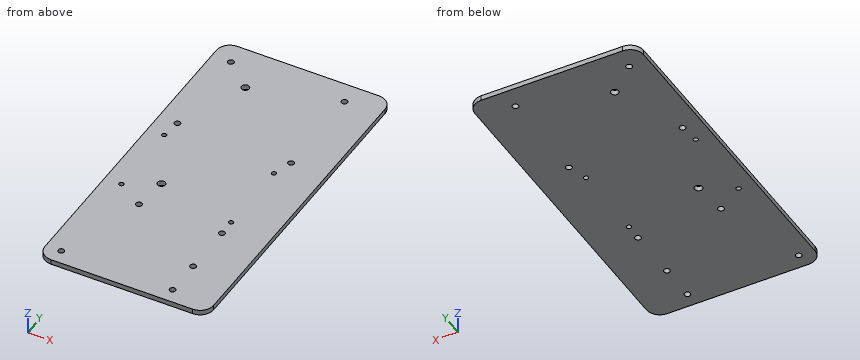
from build123d import *

# Parameters (mm, degrees)
CYLINDER_R        = 1.8
CYLINDER_DEPTH    = 10
CYLINDER002_R     = 2.3
CYLINDER002_DEPTH = 20
ARRAY001_Y_COUNT  = 2
ARRAY001_Y_PITCH  = 90
CYLINDER001_R     = 1.4
CYLINDER001_DEPTH = 10
ARRAY_X_COUNT     = 2
ARRAY_X_PITCH     = 65
ARRAY_Y_COUNT     = 2
ARRAY_Y_PITCH     = 46
CYLINDER011_R     = 1.8
CYLINDER011_DEPTH = 20
ARRAY007_X_COUNT  = 2
ARRAY007_X_PITCH  = 67.4
ARRAY007_Y_COUNT  = 2
ARRAY007_Y_PITCH  = 57.4
BOX_W             = 100
BOX_H             = 200
BOX_DEPTH         = 3
FILLET_R          = 8


with BuildPart() as m3_bolt_hole:
    # Cylinder → Cylinder (new body)
    with BuildSketch(Plane.XY):
        Circle(CYLINDER_R)
    extrude(amount=CYLINDER_DEPTH)


with BuildPart() as m3_bolt_hole_clone003:
    # Body003 base: copy of m3 bolt hole
    add(m3_bolt_hole.part)


with BuildPart() as m3_bolt_hole_clone003_1:
    # Body003 placement: moved
    add(m3_bolt_hole_clone003.part.moved(Location((30.2, -3.5, 0))))


with BuildPart() as m3_bolt_hole_clone002:
    # Body002 base: copy of m3 bolt hole
    add(m3_bolt_hole.part)


with BuildPart() as m3_bolt_hole_clone002_1:
    # Body002 placement: moved
    add(m3_bolt_hole_clone002.part.moved(Location((30.2, 27.5, 0))))


with BuildPart() as m3_bolt_hole_clone001:
    # Body001 base: copy of m3 bolt hole
    add(m3_bolt_hole.part)


with BuildPart() as m3_bolt_hole_clone001_1:
    # Body001 placement: moved
    add(m3_bolt_hole_clone001.part.moved(Location((-35.8, -25.5, 0))))


with BuildPart() as m3_bolt_hole_clone:
    # Body base: copy of m3 bolt hole
    add(m3_bolt_hole.part)


with BuildPart() as m3_bolt_hole_clone_1:
    # Body placement: moved
    add(m3_bolt_hole_clone.part.moved(Location((-19, 27.5, 0))))


with BuildPart() as attach_m4_bolt_array:
    # Cylinder002 → Cylinder002 (new body)
    with BuildSketch(Plane.XY):
        Circle(CYLINDER002_R)
    extrude(amount=CYLINDER002_DEPTH)

    # Array001 Y: attach m4 bolt array ×2


with BuildPart() as attach_m4_bolt_array_1:
    add(attach_m4_bolt_array.part)
    with Locations(*[(0, i * ARRAY001_Y_PITCH, 0) for i in range(1, ARRAY001_Y_COUNT)]):
        add(attach_m4_bolt_array.part)


with BuildPart() as attach_m4_bolt_array_2:
    # Array001 placement: moved
    add(attach_m4_bolt_array_1.part.moved(Location((-17, 48, -6))))


with BuildPart() as m2_5_bolt_hole_7x5_pcb_array:
    # Cylinder001 → Cylinder001 (new body)
    with BuildSketch(Plane.XY):
        Circle(CYLINDER001_R)
    extrude(amount=CYLINDER001_DEPTH)

    # Array X: m2.5 bolt hole 7x5 pcb array ×2


with BuildPart() as m2_5_bolt_hole_7x5_pcb_array_1:
    add(m2_5_bolt_hole_7x5_pcb_array.part)
    with Locations(*[(i * ARRAY_X_PITCH, 0, 0) for i in range(1, ARRAY_X_COUNT)]):
        add(m2_5_bolt_hole_7x5_pcb_array.part)

    # Array Y: m2.5 bolt hole 7x5 pcb array ×2


with BuildPart() as m2_5_bolt_hole_7x5_pcb_array_2:
    add(m2_5_bolt_hole_7x5_pcb_array_1.part)
    with Locations(*[(0, i * ARRAY_Y_PITCH, 0) for i in range(1, ARRAY_Y_COUNT)]):
        add(m2_5_bolt_hole_7x5_pcb_array_1.part)


with BuildPart() as m2_5_bolt_hole_7x5_pcb_array_3:
    # Array placement: moved
    add(m2_5_bolt_hole_7x5_pcb_array_2.part.moved(Location((-35, 37.6, 0))))


with BuildPart() as wall_box_hole_stand_array002:
    # Cylinder011 → Cylinder011 (new body)
    with BuildSketch(Plane(origin=(3.3, 3.3, 0), x_dir=(1, 0, 0), z_dir=(0, 0, 1))):
        Circle(CYLINDER011_R)
    extrude(amount=CYLINDER011_DEPTH)

    # Array007 X: wall box hole stand array002 ×2


with BuildPart() as wall_box_hole_stand_array002_1:
    add(wall_box_hole_stand_array002.part)
    with Locations(*[(i * ARRAY007_X_PITCH, 0, 0) for i in range(1, ARRAY007_X_COUNT)]):
        add(wall_box_hole_stand_array002.part)

    # Array007 Y: wall box hole stand array002 ×2


with BuildPart() as wall_box_hole_stand_array002_2:
    add(wall_box_hole_stand_array002_1.part)
    with Locations(*[(0, i * ARRAY007_Y_PITCH, 0) for i in range(1, ARRAY007_Y_COUNT)]):
        add(wall_box_hole_stand_array002_1.part)


with BuildPart() as wall_box_hole_stand_array002_3:
    # Array007 placement: moved
    add(wall_box_hole_stand_array002_2.part.moved(Location((-37, 92, -6))))


with BuildPart() as cnc_v4_m3_hole_fusion:
    # Body004 base: copy of m3 bolt hole
    add(m3_bolt_hole.part)


with BuildPart() as cnc_v4_m3_hole_fusion_1:
    # Body004 placement: moved
    add(cnc_v4_m3_hole_fusion.part.moved(Location((30.2, -25.5, 0))))

    # Fusion: union m3 bolt hole clone003, m3 bolt hole clone002, m3 bolt hole clone001, m3 bolt hole clone, attach m4 bolt array, m2.5 bolt hole 7x5 pcb array, wall box hole stand array002
    add(m3_bolt_hole_clone003_1.part)
    add(m3_bolt_hole_clone002_1.part)
    add(m3_bolt_hole_clone001_1.part)
    add(m3_bolt_hole_clone_1.part)
    add(attach_m4_bolt_array_2.part)
    add(m2_5_bolt_hole_7x5_pcb_array_3.part)
    add(wall_box_hole_stand_array002_3.part)


with BuildPart() as cnc_v4_m3_hole_fusion_2:
    # Fusion placement: moved
    add(cnc_v4_m3_hole_fusion_1.part.moved(Location((45, 34.4, -2.25))))


with BuildPart() as cnc_v4_plate_cut:
    # Box → Box (new body)
    with BuildSketch(Plane.XY):
        with Locations((50, 100)):
            Rectangle(BOX_W, BOX_H)
    extrude(amount=BOX_DEPTH)

    # Fillet
    fillet_edges = [cnc_v4_plate_cut.edges().sort_by_distance(p)[0] for p in [
        (0, 0, 1.5),
        (0, 200, 1.5),
        (100, 0, 1.5),
        (100, 200, 1.5),
    ]]
    fillet(fillet_edges, radius=FILLET_R)

    # Cut008: cut cnc v4 m3 hole fusion
    add(cnc_v4_m3_hole_fusion_2.part, mode=Mode.SUBTRACT)


solid = cnc_v4_plate_cut.part
Model file for the job. Use its own axes, mm. Give positions to 0.01 mm unless a question says otherwise; leave off trailing zeros. Loops run counter-clockwise (first coordinate to the right, second up) from the corner with the lowest first, then second, coordinate; pieces in that order, holes last. Notation, with made-up numbers: (26, 52.25) -> (36, 52.25) arc R21 cw to (36, 60.25) -> close; hole circle Ø4 at (11.25, 86.25). An arc over 180 degrees is marked (long way). Use a Markdown table: item, result. Add a question column.
(1) Slice it at A-A on y = 61.9. List the corners of the cut face in (x, z).
(2) Wall check: line 1 along Y through (x, z) = (28, 1.65); line 2 along X through (y, z) = (62, 1.15); line 3 along X through (y, z) = (187.5, 2.4) (3 decimals). Give the ranges that are in metal, low to high.
(3) Drop a flat-ended pin along its axis: pin 1 Ø6 at (x, y) = (78.7, 129.7) entering from -Z. Give the stop position or say it passes through.
Filled sheet:
| question | item | result |
|---|---|---|
| 1 | outline | (0, 0) -> (24.2, 0) -> (24.2, 3) -> (0, 3) -> close; (27.8, 0) -> (73.4, 0) -> (73.4, 3) -> (27.8, 3) -> close; (77, 0) -> (100, 0) -> (100, 3) -> (77, 3) -> close |
| 2 | line 1 | 0 to 80.1, 84.7 to 170.1, 174.7 to 200 |
| 2 | line 2 | 0 to 24.2, 27.8 to 73.4, 77 to 100 |
| 2 | line 3 | 0 to 9.545, 13.055 to 76.945, 80.455 to 100 |
| 3 | pin 1 | z = 0 |
